Part model, mm, in its own coordinate system. A direction names the side the tool comes from. Give positions to 0.01 mm unless a question says otherwise; leave off trailing zeros. Order: outer loops, then holes, each group sorted by start corner. A loop starts at its lowest first (then second) coordinate and runs counter-clockwise, first axis right, second up. Notation, with made-up numbers: M 56.25,19 L 100.25,19 A28 ccw 100.25,43 Z; hole C 40,7 d7. An arc over 180 degrees is marked long. Return JSON: item names as keys, results as strings.
from build123d import *

# Parameters (mm, degrees)
SKETCH_1_R          = 1
SKETCH_1_W          = 21
SKETCH_1_H          = 14
EXTRUDE_1_DEPTH     = 3
CHAMFER_1_SIZE      = 2
FILLET_2_R          = 1
SKETCH_11_R         = 1
CUT_EXTRUDE_1_DEPTH = 33.992893462


with BuildPart() as part:
    # 草图1 → 凸台-拉伸1 (new body)
    with BuildSketch(Plane.XY):
        Polygon((-21.428351104, 24.906962627), (19.571648896, 24.906962627), (19.571648896, -9.093037373), (17.69677195, -9.093037373), (15.571648896, -9.093037373), (13.89965532, -7.493037373), (-15.756357529, -7.493037373), (-17.428351104, -9.093037373), (-21.428351104, -9.093037373), align=None)
        with Locations((-12.428351104, 18.906962627)):
            Circle(SKETCH_1_R, mode=Mode.SUBTRACT)
        with Locations((-12.428351104, -4.893037373)):
            Circle(SKETCH_1_R, mode=Mode.SUBTRACT)
        with Locations((10.571648896, 18.906962627)):
            Circle(SKETCH_1_R, mode=Mode.SUBTRACT)
        with Locations((10.571648896, -4.893037373)):
            Circle(SKETCH_1_R, mode=Mode.SUBTRACT)
        with Locations((-0.928351104, 7.906962627)):
            Rectangle(SKETCH_1_W, SKETCH_1_H, mode=Mode.SUBTRACT)
    extrude(amount=EXTRUDE_1_DEPTH)

    # 倒角1
    chamfer_1_edges = [part.edges().sort_by_distance(p)[0] for p in [
        (-11.428351104, 7.906962627, 3),
        (-0.928351104, 0.906962627, 3),
        (9.571648896, 7.906962627, 3),
        (-0.928351104, 14.906962627, 3),
    ]]
    chamfer(chamfer_1_edges, length=CHAMFER_1_SIZE)

    # 圆角2
    fillet_2_edges = [part.edges().sort_by_distance(p)[0] for p in [
        (-16.592354317, -8.293037373, 3),
        (-0.928351104, -7.493037373, 3),
        (14.735652108, -8.293037373, 3),
        (17.571648896, -9.093037373, 3),
        (19.571648896, 7.906962627, 3),
        (-0.928351104, 24.906962627, 3),
        (-21.428351104, 7.906962627, 3),
        (-19.428351104, -9.093037373, 3),
    ]]
    fillet(fillet_2_edges, radius=FILLET_2_R)

    # 草图11 → 切除-拉伸1 (cut, through all)
    with BuildSketch(Plane.XY.offset(3)):
        with Locations((-18.428351104, 21.906962627)):
            Circle(SKETCH_11_R)
        with Locations((-18.428351104, -4.093037373)):
            Circle(SKETCH_11_R)
        with Locations((16.571648896, 21.906962627)):
            Circle(SKETCH_11_R)
        with Locations((16.571648896, -4.093037373)):
            Circle(SKETCH_11_R)
    extrude(amount=-CUT_EXTRUDE_1_DEPTH, mode=Mode.SUBTRACT)


solid = part.part
Q1. Pin check, flat tips, straight feed: pin 1 (1.2 mm diameter, centred on x = -12.43, y = -4.89, fed in from +Z); pin 2 (1.6 mm diameter, centred on x = 2, z = 1.5, fed in from -Y); pin 3 (8 mm diameter, centred on x = -8, y = 10.5, fed in from +Z). Stop position of each tip, or through.
Established:
{"pin 1": "passes through", "pin 2": "stops at y = -7.49", "pin 3": "stops at z = 1.57"}
Q2. 3-axis set-ups, long thin cutter, end or side, ignore diameter. For faces 1 (the flat face through (-1, -7.493, 1)), 2 (the cylindrical face through (-0.64, 24.61, 2.71)), 3 (the cylindrical face through (-21.13, 8.14, 2.71)), 4 (the flat face through (-11.428, 7.8, 0.5)), 5 (the cylindrical face through (-1.142, -7.192, 2.715)): which of +Z, -Z, +X, -X, +Y, -Y reach the whole face in a straight line?
Established:
{"face 1": "+Z, -Z, -Y", "face 2": "+Z, +X, -X, +Y", "face 3": "+Z, -X, +Y, -Y", "face 4": "+Z, -Z", "face 5": "+Z, -Y"}
Q3. Band-saw the part on A-A (x = 3.5). Give the cut face in (y, z), then the cut area to 3 significant figures.
Established:
{"outline": "M -7.49,0 L 0.91,0 L 0.91,1 L -1.09,3 L -6.49,3 A1 ccw -7.49,2 Z; M 14.91,0 L 24.91,0 L 24.91,2 A1 ccw 23.91,3 L 16.91,3 L 14.91,1 Z", "area": "50.8 mm²"}
Q4. Probe line 1 along X through (y, z) = (13, 0.2); line 2 along X through (y, z) = (18.5, 0.7); line 3 along Y through (x, z) = (-6.5, 0.4). List the from-to ranges inside material, lowest first.
Established:
{"line 1": "x = -21.43 to -11.43, 9.57 to 19.57", "line 2": "x = -21.43 to -13.34, -11.51 to 9.66, 11.49 to 19.57", "line 3": "y = -7.49 to 0.91, 14.91 to 24.91"}
Q5. Band-saw the part on B-B (x = -12.5). Give the cut face in (y, z), then the cut area to 3 significant figures.
Established:
{"outline": "M -7.49,0 L -5.89,0 L -5.89,3 L -6.49,3 A1 ccw -7.49,2 Z; M -3.9,0 L 17.91,0 L 17.91,3 L 16.91,3 L 15.98,2.07 L -0.16,2.07 L -1.09,3 L -3.9,3 Z; M 19.9,0 L 24.91,0 L 24.91,2 A1 ccw 23.91,3 L 19.9,3 Z", "area": "69.0 mm²"}
Q6. Two-plate mould, pull along X, no slides. Class faces 6 (the flat face through (18, -9.093, 1)), 7 (the flat face through (-21.428, 8, 1)), 8 (the flat face through (14.747, -8.304, 0.986)), 9 (the cylindrical face through (19.271, 7.669, 2.715)): +X half, -X half, draft (parallel to the pull), parting line (faces both ways), or undercut.
Established:
{"face 6": "draft", "face 7": "-X half", "face 8": "undercut", "face 9": "+X half"}
Q7. Band-saw the part on C-C (z = 2.5). Give the number of separate pieces and of enclosed holes in the cut face, then the cut area to 3 significant figures.
Established:
{"separate pieces": "1", "enclosed holes": "9", "area": "891 mm²"}
